```python
from build123d import *

# Parameters (mm, degrees)
BOSS_EXTRUDE1_DEPTH = 1219.2
FILLET1_R           = 0.254
SKETCH4_W           = 1838.4
SKETCH4_H           = 74.945320812
CUT_EXTRUDE1_DEPTH  = 60
SKETCH5_R           = 1.65
CUT_EXTRUDE2_DEPTH  = 10
SKETCH9_R           = 1.65
CUT_EXTRUDE6_DEPTH  = 60


with BuildPart() as part:
    # Sketch3 → Boss-Extrude1 (new, symmetric)
    with BuildSketch(Plane.XY):
        Polygon((1.5875, 25.4), (0, 25.4), (0, 0), (25.4, 0), (25.4, 1.5875), (1.5875, 1.5875), align=None)
    extrude(amount=BOSS_EXTRUDE1_DEPTH, both=True)

    # Fillet1
    fillet1_edges = [part.edges().sort_by_distance(p)[0] for p in [
        (1.5875, 1.5875, 0),
    ]]
    fillet(fillet1_edges, radius=FILLET1_R)

    # Sketch4 → Cut-Extrude1 (cut)
    with BuildSketch(Plane.ZY):
        with Locations((-300, 37.472660406)):
            Rectangle(SKETCH4_W, SKETCH4_H)
    extrude(amount=-CUT_EXTRUDE1_DEPTH, mode=Mode.SUBTRACT)

    # Sketch5 → Cut-Extrude2 (cut)
    with BuildSketch(Plane(origin=(0, 1.5875, 0), x_dir=(1, 0, 0), z_dir=(0, 1, 0))):
        with Locations(Location((17.4625, -629.5759, 0), (0, 0, 180))):
            Circle(SKETCH5_R)
        with Locations(Location((17.4625, -1208.8241, 0), (0, 0, 180))):
            Circle(SKETCH5_R)
        with Locations(Location((13.49375, -1189.2, 0), (0, 0, 180))):
            Circle(SKETCH5_R)
        with Locations(Location((13.49375, -1169.2, 0), (0, 0, 180))):
            Circle(SKETCH5_R)
        with Locations(Location((13.49375, -1149.2, 0), (0, 0, 180))):
            Circle(SKETCH5_R)
        with Locations(Location((13.49375, -1129.2, 0), (0, 0, 180))):
            Circle(SKETCH5_R)
        with Locations(Location((13.49375, -1109.2, 0), (0, 0, 180))):
            Circle(SKETCH5_R)
        with Locations(Location((13.49375, -1089.2, 0), (0, 0, 180))):
            Circle(SKETCH5_R)
        with Locations(Location((13.49375, -1069.2, 0), (0, 0, 180))):
            Circle(SKETCH5_R)
        with Locations(Location((13.49375, -1049.2, 0), (0, 0, 180))):
            Circle(SKETCH5_R)
        with Locations(Location((13.49375, -1029.2, 0), (0, 0, 180))):
            Circle(SKETCH5_R)
        with Locations(Location((13.49375, -1009.2, 0), (0, 0, 180))):
            Circle(SKETCH5_R)
        with Locations(Location((13.49375, -989.2, 0), (0, 0, 180))):
            Circle(SKETCH5_R)
        with Locations(Location((13.49375, -969.2, 0), (0, 0, 180))):
            Circle(SKETCH5_R)
        with Locations(Location((13.49375, -949.2, 0), (0, 0, 180))):
            Circle(SKETCH5_R)
        with Locations(Location((13.49375, -929.2, 0), (0, 0, 180))):
            Circle(SKETCH5_R)
        with Locations(Location((13.49375, -909.2, 0), (0, 0, 180))):
            Circle(SKETCH5_R)
        with Locations(Location((13.49375, -889.2, 0), (0, 0, 180))):
            Circle(SKETCH5_R)
        with Locations(Location((13.49375, -869.2, 0), (0, 0, 180))):
            Circle(SKETCH5_R)
        with Locations(Location((13.49375, -849.2, 0), (0, 0, 180))):
            Circle(SKETCH5_R)
        with Locations(Location((13.49375, -829.2, 0), (0, 0, 180))):
            Circle(SKETCH5_R)
        with Locations(Location((13.49375, -809.2, 0), (0, 0, 180))):
            Circle(SKETCH5_R)
        with Locations(Location((13.49375, -789.2, 0), (0, 0, 180))):
            Circle(SKETCH5_R)
        with Locations(Location((13.49375, -769.2, 0), (0, 0, 180))):
            Circle(SKETCH5_R)
        with Locations(Location((13.49375, -749.2, 0), (0, 0, 180))):
            Circle(SKETCH5_R)
        with Locations(Location((13.49375, -729.2, 0), (0, 0, 180))):
            Circle(SKETCH5_R)
        with Locations(Location((13.49375, -709.2, 0), (0, 0, 180))):
            Circle(SKETCH5_R)
        with Locations(Location((13.49375, -689.2, 0), (0, 0, 180))):
            Circle(SKETCH5_R)
        with Locations(Location((13.49375, -669.2, 0), (0, 0, 180))):
            Circle(SKETCH5_R)
        with Locations(Location((13.49375, -649.2, 0), (0, 0, 180))):
            Circle(SKETCH5_R)
    extrude(amount=-CUT_EXTRUDE2_DEPTH, mode=Mode.SUBTRACT)

    # Sketch9 → Cut-Extrude6 (cut)
    with BuildSketch(Plane(origin=(1.5875, 0, 0), x_dir=(0, 0, -1), z_dir=(1, 0, 0))):
        with Locations((-629.5759, 17.4625)):
            Circle(SKETCH9_R)
        with Locations((-1208.8241, 17.463)):
            Circle(SKETCH9_R)
        with Locations((-1188.258925, 13.49375)):
            Circle(SKETCH9_R)
        with Locations((-1168.258925, 13.49375)):
            Circle(SKETCH9_R)
        with Locations((-1148.258925, 13.49375)):
            Circle(SKETCH9_R)
        with Locations((-1128.258925, 13.49375)):
            Circle(SKETCH9_R)
        with Locations((-1108.258925, 13.49375)):
            Circle(SKETCH9_R)
        with Locations((-1088.258925, 13.49375)):
            Circle(SKETCH9_R)
        with Locations((-1068.258925, 13.49375)):
            Circle(SKETCH9_R)
        with Locations((-1048.258925, 13.49375)):
            Circle(SKETCH9_R)
        with Locations((-1028.258925, 13.49375)):
            Circle(SKETCH9_R)
        with Locations((-1008.258925, 13.49375)):
            Circle(SKETCH9_R)
        with Locations((-988.258925, 13.49375)):
            Circle(SKETCH9_R)
        with Locations((-968.258925, 13.49375)):
            Circle(SKETCH9_R)
        with Locations((-948.258925, 13.49375)):
            Circle(SKETCH9_R)
        with Locations((-928.258925, 13.49375)):
            Circle(SKETCH9_R)
        with Locations((-787.69375, 14.2875)):
            Circle(SKETCH9_R)
        with Locations((-907.69375, 14.2875)):
            Circle(SKETCH9_R)
        with Locations((-648.634825, 13.49375)):
            Circle(SKETCH9_R)
        with Locations((-668.634825, 13.49375)):
            Circle(SKETCH9_R)
        with Locations((-688.634825, 13.49375)):
            Circle(SKETCH9_R)
        with Locations((-708.634825, 13.49375)):
            Circle(SKETCH9_R)
        with Locations((-728.634825, 13.49375)):
            Circle(SKETCH9_R)
        with Locations((-748.634825, 13.49375)):
            Circle(SKETCH9_R)
        with Locations((-768.634825, 13.49375)):
            Circle(SKETCH9_R)
        with Locations((-808.634825, 13.49375)):
            Circle(SKETCH9_R)
        with Locations((-828.634825, 13.49375)):
            Circle(SKETCH9_R)
        with Locations((-848.634825, 13.49375)):
            Circle(SKETCH9_R)
        with Locations((-868.634825, 13.49375)):
            Circle(SKETCH9_R)
        with Locations((-888.634825, 13.49375)):
            Circle(SKETCH9_R)
    extrude(amount=-CUT_EXTRUDE6_DEPTH, mode=Mode.SUBTRACT)


solid = part.part
```
Verification items for the finished model (mm, model axes). A direction names the side the tool comes from. Coordinates: 2 decimals unless noted, no trailing zeros. Loops run counter-clockwise (first coordinate to the right, second up) from the corner with the lowest first, then second, coordinate; pieces in that order, holes last. Notation, with made-up numbers: (18, 3) -> (23, 3) arc R23 ccw to (23, 26) -> close; hole circle Ø4 at (30, -2.75). An arc over 180 degrees is marked (long way). Answer in a Markdown table with one row per item.
1) Section check A-A (z = 936.5). Record the cut outline in (x, y).
The answers:
| item | result |
|---|---|
| outline | (0, 0) -> (25.4, 0) -> (25.4, 1.59) -> (1.84, 1.59) arc R0.25 cw to (1.59, 1.84) -> (1.59, 25.4) -> (0, 25.4) -> close |
2) Depth check by flat-ended pin: P1, Ø5.5, axis at x = 13.49, z = 1169.2, coming from the +Y side; P2, Ø2, axis at y = 11.5, z = 963.5, coming from the +X side; P3, Ø3, axis at x = 13.49, z = 809.2, coming from the +Y side. Enter the tip coordinate at first touch or a pass-through.
The answers:
| item | result |
|---|---|
| P1 | stops at y = 1.59 |
| P2 | stops at x = 1.59 |
| P3 | passes through |
3) Access from +Z, -Z, +X, -X, +Y, -Y to the whole of each face (thin tool, end or side, straight path). Record for faces 1 (the face through (14, 1.588, 923)), 2 (the face through (0, 13, 923)).
The answers:
| item | result |
|---|---|
| face 1 | +Z, -Z, +X, +Y |
| face 2 | +Z, -Z, -X, +Y, -Y |
4) Section check B-B (x = 7). Record the cut outline in (y, z).
The answers:
| item | result |
|---|---|
| outline | (0, 619.2) -> (1.59, 619.2) -> (1.59, 1219.2) -> (0, 1219.2) -> close |
5) Scan lines: line 1 along X through (y, z) = (0.55, 1129.2); line 2 along X through (y, z) = (16.25, 682). Record each from-to range of solid material in increasing order. Write a range as from..to.
The answers:
| item | result |
|---|---|
| line 1 | x = 0..11.84, 15.14..25.4 |
| line 2 | x = 0..1.59 |
